```python
from build123d import *

# Parameters (mm, degrees)
SKETCH1_R           = 15
SKETCH1_R_2         = 2.25
BOSS_EXTRUDE2_DEPTH = 10


with BuildPart() as part:
    # Sketch1 → Boss-Extrude2 (new body)
    with BuildSketch(Plane(origin=(0, 0, 0), x_dir=(0, 0, -1), z_dir=(1, 0, 0))):
        with BuildLine():
            ThreePointArc((12.720721442, 7.948788963), (13.481910694, 6.575567202), (14.095389312, 5.13030215))
            Line((14.095389312, 5.13030215), (14.565235622, 5.301312222))
            ThreePointArc((14.565235622, 5.301312222), (18.908034497, 7.529506054), (22.564632109, 10.76277742))
            Line((22.564632109, 10.76277742), (22.469851157, 10.95927867))
            Line((22.469851157, 10.95927867), (22.37335904, 11.154945328))
            ThreePointArc((22.37335904, 11.154945328), (17.574280154, 10.264107707), (13.14474549, 8.213748596))
            Line((13.14474549, 8.213748596), (12.720721442, 7.948788963))
        make_face()
        with BuildLine():
            ThreePointArc((9.23492213, 11.820161304), (10.419875557, 10.790097005), (11.490666647, 9.641814145))
            Line((11.490666647, 9.641814145), (11.873688868, 9.96320795))
            ThreePointArc((11.873688868, 9.96320795), (15.19249775, 13.542349946), (17.522731607, 17.831261229))
            Line((17.522731607, 17.831261229), (17.366459261, 17.983495008))
            Line((17.366459261, 17.983495008), (17.208864392, 18.134359275))
            ThreePointArc((17.208864392, 18.134359275), (13.003889787, 15.655864088), (9.542752868, 12.214166681))
            Line((9.542752868, 12.214166681), (9.23492213, 11.820161304))
        make_face()
        with BuildLine():
            ThreePointArc((4.635254916, 14.265847744), (6.101049646, 13.703181865), (7.5, 12.990381057))
            Line((7.5, 12.990381057), (7.75, 13.423393759))
            ThreePointArc((7.75, 13.423393759), (9.644521558, 17.92178657), (10.367331066, 22.749031772))
            Line((10.367331066, 22.749031772), (10.168416077, 22.838636441))
            Line((10.168416077, 22.838636441), (9.968726723, 22.92650186))
            ThreePointArc((9.968726723, 22.92650186), (6.865038395, 19.159292205), (4.789763413, 14.741376003))
            Line((4.789763413, 14.741376003), (4.635254916, 14.265847744))
        make_face()
        with BuildLine():
            ThreePointArc((-0.523492451, 14.990862405), (1.046347106, 14.963460754), (2.604722665, 14.772116295))
            Line((2.604722665, 14.772116295), (2.691546754, 15.264520172))
            ThreePointArc((2.691546754, 15.264520172), (2.933273727, 20.139591237), (1.961477393, 24.922933343))
            Line((1.961477393, 24.922933343), (1.743911844, 24.939101256))
            Line((1.743911844, 24.939101256), (1.526213488, 24.953369961))
            ThreePointArc((1.526213488, 24.953369961), (-0.101837945, 20.35182692), (-0.540942199, 15.490557819))
            Line((-0.540942199, 15.490557819), (-0.523492451, 14.990862405))
        make_face()
        with BuildLine():
            ThreePointArc((-5.619098901, 13.907757819), (-4.134560337, 14.418925439), (-2.604722665, 14.772116295))
            Line((-2.604722665, 14.772116295), (-2.691546754, 15.264520172))
            ThreePointArc((-2.691546754, 15.264520172), (-4.131770205, 19.928263972), (-6.680959402, 24.09076133))
            Line((-6.680959402, 24.09076133), (-6.890933895, 24.031542398))
            Line((-6.890933895, 24.031542398), (-7.100383618, 23.970493372))
            ThreePointArc((-7.100383618, 23.970493372), (-7.056431125, 19.089630948), (-5.806402198, 14.371349746))
            Line((-5.806402198, 14.371349746), (-5.619098901, 13.907757819))
        make_face()
        with BuildLine():
            ThreePointArc((-10.036959095, 11.147172382), (-8.816778784, 12.135254916), (-7.5, 12.990381057))
            Line((-7.5, 12.990381057), (-7.75, 13.423393759))
            ThreePointArc((-7.75, 13.423393759), (-10.698461672, 17.313293962), (-14.517573893, 20.352887959))
            Line((-14.517573893, 20.352887959), (-14.694631307, 20.225424859))
            Line((-14.694631307, 20.225424859), (-14.870569669, 20.096421515))
            ThreePointArc((-14.870569669, 20.096421515), (-13.15991457, 15.524943751), (-10.371524399, 11.518744795))
            Line((-10.371524399, 11.518744795), (-10.036959095, 11.147172382))
        make_face()
        with BuildLine():
            ThreePointArc((-13.244213893, 7.042073442), (-12.435563588, 8.387893552), (-11.490666647, 9.641814145))
            Line((-11.490666647, 9.641814145), (-11.873688868, 9.96320795))
            ThreePointArc((-11.873688868, 9.96320795), (-15.974760769, 12.610085183), (-20.603154716, 14.160155923))
            Line((-20.603154716, 14.160155923), (-20.725939314, 13.979822587))
            Line((-20.725939314, 13.979822587), (-20.847145552, 13.798424633))
            ThreePointArc((-20.847145552, 13.798424633), (-17.676118098, 10.087719213), (-13.685687689, 7.276809223))
            Line((-13.685687689, 7.276809223), (-13.244213893, 7.042073442))
        make_face()
        with BuildLine():
            ThreePointArc((-14.854021031, 2.087596514), (-14.554435894, 3.628828434), (-14.095389312, 5.13030215))
            Line((-14.095389312, 5.13030215), (-14.565235622, 5.301312222))
            ThreePointArc((-14.565235622, 5.301312222), (-19.324267955, 6.385914026), (-24.203691009, 6.259500101))
            Line((-24.203691009, 6.259500101), (-24.257393157, 6.04804739))
            Line((-24.257393157, 6.04804739), (-24.30924801, 5.836134096))
            ThreePointArc((-24.30924801, 5.836134096), (-20.060320912, 3.43376686), (-15.349155065, 2.157183065))
            Line((-15.349155065, 2.157183065), (-14.854021031, 2.087596514))
        make_face()
        with BuildLine():
            Line((-15.161287811, -3.222631208), (-14.672214011, -3.118675362))
            ThreePointArc((-14.672214011, -3.118675362), (-14.917828431, -1.567926949), (-15, 0))
            Line((-15, 0), (-15.5, 0))
            ThreePointArc((-15.5, 0), (-20.34298323, -0.608492609), (-24.884904959, -2.396143813))
            Line((-24.884904959, -2.396143813), (-24.863047384, -2.613211582))
            Line((-24.863047384, -2.613211582), (-24.839296392, -2.830080344))
            ThreePointArc((-24.839296392, -2.830080344), (-20.024952965, -3.634348454), (-15.161287811, -3.222631208))
        make_face()
        with BuildLine():
            Line((-13.14474549, -8.213748596), (-12.720721442, -7.948788963))
            ThreePointArc((-12.720721442, -7.948788963), (-13.481910694, -6.575567202), (-14.095389312, -5.13030215))
            Line((-14.095389312, -5.13030215), (-14.565235622, -5.301312222))
            ThreePointArc((-14.565235622, -5.301312222), (-18.908034497, -7.529506054), (-22.564632109, -10.76277742))
            Line((-22.564632109, -10.76277742), (-22.469851157, -10.95927867))
            Line((-22.469851157, -10.95927867), (-22.37335904, -11.154945328))
            ThreePointArc((-22.37335904, -11.154945328), (-17.574280154, -10.264107707), (-13.14474549, -8.213748596))
        make_face()
        with BuildLine():
            Line((-9.542752868, -12.214166681), (-9.23492213, -11.820161304))
            ThreePointArc((-9.23492213, -11.820161304), (-10.419875557, -10.790097005), (-11.490666647, -9.641814145))
            Line((-11.490666647, -9.641814145), (-11.873688868, -9.96320795))
            ThreePointArc((-11.873688868, -9.96320795), (-15.19249775, -13.542349946), (-17.522731607, -17.831261229))
            Line((-17.522731607, -17.831261229), (-17.366459261, -17.983495008))
            Line((-17.366459261, -17.983495008), (-17.208864392, -18.134359275))
            ThreePointArc((-17.208864392, -18.134359275), (-13.003889787, -15.655864088), (-9.542752868, -12.214166681))
        make_face()
        with BuildLine():
            Line((-4.789763413, -14.741376003), (-4.635254916, -14.265847744))
            ThreePointArc((-4.635254916, -14.265847744), (-6.101049646, -13.703181865), (-7.5, -12.990381057))
            Line((-7.5, -12.990381057), (-7.75, -13.423393759))
            ThreePointArc((-7.75, -13.423393759), (-9.644521558, -17.92178657), (-10.367331066, -22.749031772))
            Line((-10.367331066, -22.749031772), (-10.168416077, -22.838636441))
            Line((-10.168416077, -22.838636441), (-9.968726723, -22.92650186))
            ThreePointArc((-9.968726723, -22.92650186), (-6.865038395, -19.159292205), (-4.789763413, -14.741376003))
        make_face()
        with BuildLine():
            Line((0.540942199, -15.490557819), (0.523492451, -14.990862405))
            ThreePointArc((0.523492451, -14.990862405), (-1.046347106, -14.963460754), (-2.604722665, -14.772116295))
            Line((-2.604722665, -14.772116295), (-2.691546754, -15.264520172))
            ThreePointArc((-2.691546754, -15.264520172), (-2.933273727, -20.139591237), (-1.961477393, -24.922933343))
            Line((-1.961477393, -24.922933343), (-1.743911844, -24.939101256))
            Line((-1.743911844, -24.939101256), (-1.526213488, -24.953369961))
            ThreePointArc((-1.526213488, -24.953369961), (0.101837945, -20.35182692), (0.540942199, -15.490557819))
        make_face()
        with BuildLine():
            Line((5.806402198, -14.371349746), (5.619098901, -13.907757819))
            ThreePointArc((5.619098901, -13.907757819), (4.134560337, -14.418925439), (2.604722665, -14.772116295))
            Line((2.604722665, -14.772116295), (2.691546754, -15.264520172))
            ThreePointArc((2.691546754, -15.264520172), (4.131770205, -19.928263972), (6.680959402, -24.09076133))
            Line((6.680959402, -24.09076133), (6.890933895, -24.031542398))
            Line((6.890933895, -24.031542398), (7.100383618, -23.970493372))
            ThreePointArc((7.100383618, -23.970493372), (7.056431125, -19.089630948), (5.806402198, -14.371349746))
        make_face()
        with BuildLine():
            Line((10.371524399, -11.518744795), (10.036959095, -11.147172382))
            ThreePointArc((10.036959095, -11.147172382), (8.816778784, -12.135254916), (7.5, -12.990381057))
            Line((7.5, -12.990381057), (7.75, -13.423393759))
            ThreePointArc((7.75, -13.423393759), (10.698461672, -17.313293962), (14.517573893, -20.352887959))
            Line((14.517573893, -20.352887959), (14.694631307, -20.225424859))
            Line((14.694631307, -20.225424859), (14.870569669, -20.096421515))
            ThreePointArc((14.870569669, -20.096421515), (13.15991457, -15.524943751), (10.371524399, -11.518744795))
        make_face()
        with BuildLine():
            Line((13.685687689, -7.276809223), (13.244213893, -7.042073442))
            ThreePointArc((13.244213893, -7.042073442), (12.435563588, -8.387893552), (11.490666647, -9.641814145))
            Line((11.490666647, -9.641814145), (11.873688868, -9.96320795))
            ThreePointArc((11.873688868, -9.96320795), (15.974760769, -12.610085183), (20.603154716, -14.160155923))
            Line((20.603154716, -14.160155923), (20.725939314, -13.979822587))
            Line((20.725939314, -13.979822587), (20.847145552, -13.798424633))
            ThreePointArc((20.847145552, -13.798424633), (17.676118098, -10.087719213), (13.685687689, -7.276809223))
        make_face()
        with BuildLine():
            Line((15.349155065, -2.157183065), (14.854021031, -2.087596514))
            ThreePointArc((14.854021031, -2.087596514), (14.554435894, -3.628828434), (14.095389312, -5.13030215))
            Line((14.095389312, -5.13030215), (14.565235622, -5.301312222))
            ThreePointArc((14.565235622, -5.301312222), (19.324267955, -6.385914026), (24.203691009, -6.259500101))
            Line((24.203691009, -6.259500101), (24.257393157, -6.04804739))
            Line((24.257393157, -6.04804739), (24.30924801, -5.836134096))
            ThreePointArc((24.30924801, -5.836134096), (20.060320912, -3.43376686), (15.349155065, -2.157183065))
        make_face()
        with BuildLine():
            ThreePointArc((14.672214011, 3.118675362), (14.917828431, 1.567926949), (15, 0))
            Line((15, 0), (15.5, 0))
            ThreePointArc((15.5, 0), (20.34298323, 0.608492609), (24.884904959, 2.396143813))
            Line((24.884904959, 2.396143813), (24.863047384, 2.613211582))
            Line((24.863047384, 2.613211582), (24.839296392, 2.830080344))
            ThreePointArc((24.839296392, 2.830080344), (20.024952965, 3.634348454), (15.161287811, 3.222631208))
            Line((15.161287811, 3.222631208), (14.672214011, 3.118675362))
        make_face()
        Circle(SKETCH1_R)
        Circle(SKETCH1_R_2, mode=Mode.SUBTRACT)
    extrude(amount=BOSS_EXTRUDE2_DEPTH)


solid = part.part
```
The model under review builds one solid part; all positions refer to its coordinate system, in mm. A direction names the side the tool comes from. Round coordinates to 2 decimals unless told otherwise and drop trailing zeros. Answer as a JSON object with one key per item and string values. Group by question number.
1) Mouldability with a two-part tool opening along Z and no side actions: class faces 5 (the face through (4.9, 15.6, 13.2)), 6 (the face through (4.93, -0.592, 20.277)), 7 (the face through (4.93, 17.856, -9.626)), 8 (the face through (4.93, -10.134, -17.727)) as released by +Z, released by -Z, zero draft, split by the parting line, or undercut.
2) For line 1 (Z direction, x = 5.75, y = 12); line 2 (Y direction, x = 1, z = -19); line 3 (Y direction, x = 7.5, z = -13.5), list the stretches that pass through material, from the lowest coordinate up. Write a range as [from, to].
3) For pin 1 Ø1.5 at (x, z) = (5, -6) entering from -Y; pin 2 Ø4 at (x, y) = (4.5, 11) entering from +Z; pin 3 Ø5 at (y, z) = (-7, -18) entering from +X; pin 4 Ø0.6 at (x, z) = (6.5, -15) entering from -Y, all flat-tipped, find the tip position at first contact; note any pin that passes through.
4) For faces 1 (the face through (4.93, 13.487, -15.152)), 2 (the face through (4.93, 3.46, 20.12)), 3 (the face through (4.93, -3.46, -20.12)), 4 (the face through (4.93, 17.264, 10.651)), list the 3-axis set-ups (+Z, -Z, +X, -X, +Y, -Y) from which the entire face can be reached by the end or side of a thin tool; tool diameter is ignored.
Result set:
{
 "1": {"face 5": "undercut", "face 6": "released by +Z", "face 7": "undercut", "face 8": "released by -Z"},
 "2": {"line 1": "[-13.96, -9.38], [-9, 10.79], [14.81, 19.51]", "line 2": "[-13.77, -11.41], [-6.35, -3.03], [0.32, 3.65], [7.59, 10.66]", "line 3": "[-19.69, -16.21], [-11.19, -7.18], [-6.54, 8.43], [11.49, 16.03]"},
 "3": {"pin 1": "y = -24.09", "pin 2": "z = 20.29", "pin 3": "x = 10", "pin 4": "y = -20.22"},
 "4": {"face 1": "+X, -X", "face 2": "+Z, +X, -X", "face 3": "-Z, +X, -X", "face 4": "+X, -X, +Y"}
}
